from build123d import *

# Parameters (mm, degrees)
SKETCH1_R           = 12.15
SKETCH1_R_2         = 16.15
BOSS_EXTRUDE1_DEPTH = 5.4
FILLET1_R           = 30
CHAMFER1_SIZE       = 1
SKETCH2_R           = 14.75534968
SKETCH2_R_2         = 10
SKETCH2_R_3         = 19.025242353
SKETCH2_R_4         = 14
BOSS_EXTRUDE2_DEPTH = 0.6


with BuildPart() as part:
    # Sketch1 → Boss-Extrude1 (new body)
    with BuildSketch(Plane(origin=(0, 0, 0), x_dir=(1, 0, 0), z_dir=(0, 1, 0))):
        with BuildLine():
            Line((54.45294862, -21), (63.75, -21))
            ThreePointArc((63.75, -21), (84.75, 0), (63.75, 21))
            Line((63.75, 21), (54.45294862, 21))
            ThreePointArc((54.45294862, 21), (48.447855306, 13.72835863), (39.420454068, 11))
            Line((39.420454068, 11), (-39.420454068, 11))
            ThreePointArc((-39.420454068, 11), (-48.447855306, 13.72835863), (-54.45294862, 21))
            Line((-54.45294862, 21), (-63.75, 21))
            ThreePointArc((-63.75, 21), (-84.75, 0), (-63.75, -21))
            Line((-63.75, -21), (-54.45294862, -21))
            ThreePointArc((-54.45294862, -21), (-48.447855306, -13.72835863), (-39.420454068, -11))
            Line((-39.420454068, -11), (39.420454068, -11))
            ThreePointArc((39.420454068, -11), (48.447855306, -13.72835863), (54.45294862, -21))
        make_face()
        with Locations(Location((-63.75, 0, 0), (0, 0, 90))):
            Circle(SKETCH1_R, mode=Mode.SUBTRACT)
        with Locations(Location((63.75, 0, 0), (0, 0, 90))):
            Circle(SKETCH1_R_2, mode=Mode.SUBTRACT)
    extrude(amount=BOSS_EXTRUDE1_DEPTH)

    # Fillet1
    # the kernel refuses this fillet: 30 mm, written as the material it takes off along each edge
    with BuildSketch(Plane(origin=(-54.45294862, -23.24262845, -21), x_dir=(0.5987620470660618, 0, 0.8009269698251266), z_dir=(0, 1, 0))) as fillet1_piece_1:
        with BuildLine():
            CenterArc((15.193568911, -29.102905777), FILLET1_R, 104.047021464, 29.74238235)
            Line((-5.566721516, -7.44625919), (-5.981927325, -7.013126259))
            ThreePointArc((-5.981927325, -7.013126259), (-3.26391694, -3.363872367), (-0.480556182, 0.359257228))
            Line((-0.480556182, 0.359257228), (0.145630869, 0.582058116))
            ThreePointArc((0.145630869, 0.582058116), (3.95601272, 0.11261485), (7.76639457, 0.582058116))
            Line((7.76639457, 0.582058116), (7.912025439, 0))
        make_face()
    extrude(amount=51.885256901, mode=Mode.SUBTRACT)
    with BuildSketch(Plane(origin=(54.45294862, -23.24262845, -21), x_dir=(1, 0, 0), z_dir=(0, 1, 0)), Plane(origin=(-54.45294862, -23.24262845, 21), x_dir=(-1, 0, 0), z_dir=(0, 1, 0))) as fillet1_piece_2:
        with BuildLine():
            CenterArc((14.211969714, -29.594654547), FILLET1_R, 99.429309033, 29.74238235)
            Line((-4.737420548, -6.33695456), (-5.116408354, -5.87180056))
            ThreePointArc((-5.116408354, -5.87180056), (-2.458906545, -3.101047782), (-0.55338428, 0.231874618))
            Line((-0.55338428, 0.231874618), (0, 0.6))
            ThreePointArc((0, 0.6), (4.64852569, 0.6), (9.198753014, 0.591893091))
            Line((9.198753014, 0.591893091), (9.29705138, 0))
        make_face()
    extrude(amount=51.885256901, mode=Mode.SUBTRACT)
    with BuildSketch(Plane(origin=(54.45294862, -23.24262845, 21), x_dir=(1, 0, 0), z_dir=(0, 1, 0))) as fillet1_piece_3:
        with BuildLine():
            CenterArc((14.211969714, 29.594654547), FILLET1_R, 230.828308617, 29.74238235)
            Line((-4.737420548, 6.33695456), (-5.116408354, 5.87180056))
            ThreePointArc((-5.116408354, 5.87180056), (-2.458906545, 3.101047782), (-0.55338428, -0.231874618))
            Line((-0.55338428, -0.231874618), (0, -0.6))
            ThreePointArc((0, -0.6), (4.64852569, -0.6), (9.198753014, -0.591893091))
            Line((9.198753014, -0.591893091), (9.29705138, 0))
        make_face()
    extrude(amount=51.885256901, mode=Mode.SUBTRACT)

    # Chamfer1
    # the kernel refuses this chamfer: 1 mm, written as the material it takes off along each edge
    with BuildSketch(Plane(origin=(63.75, 5.4, 0), x_dir=(-0.12235070165055995, 0, 0.9924869297908239), z_dir=(-0.9924869297908239, 0, -0.12235070165055995))) as chamfer1_piece_1:
        Polygon((21, -CHAMFER1_SIZE), (21 - CHAMFER1_SIZE, 0), (21, 0), align=None)
    revolve(axis=Axis((63.75, 5.4, 0), (0, 1, 0)), revolution_arc=194.055575488, mode=Mode.SUBTRACT)
    with BuildSketch(Plane(origin=(39.420454068, 5.4, -27.298794623), x_dir=(0.6316463420707552, 0, 0.7752566662394039), z_dir=(0.7752566662394039, 0, -0.6316463420707552))) as chamfer1_piece_2:
        Polygon((16.298794623 + CHAMFER1_SIZE, 0), (16.298794623, CHAMFER1_SIZE), (16.298794623, 0), align=None)
    revolve(axis=Axis((39.420454068, 5.4, -27.298794623), (0, -1, 0)), revolution_arc=39.171691383, mode=Mode.SUBTRACT)
    with BuildSketch(Plane(origin=(39.420454068, 5.4, -11), x_dir=(0, 0, 1), z_dir=(-1, 0, 0)), Plane(origin=(-39.420454068, 5.4, 11), x_dir=(0, 0, -1), z_dir=(1, 0, 0))) as chamfer1_piece_3:
        Polygon((CHAMFER1_SIZE, 0), (0, -CHAMFER1_SIZE), (0, 0), align=None)
    extrude(amount=78.840908135, mode=Mode.SUBTRACT)
    with BuildSketch(Plane(origin=(-39.420454068, 5.4, -27.298794623), x_dir=(0, 0, 1), z_dir=(1, 0, 0))) as chamfer1_piece_4:
        Polygon((16.298794623 + CHAMFER1_SIZE, 0), (16.298794623, CHAMFER1_SIZE), (16.298794623, 0), align=None)
    revolve(axis=Axis((-39.420454068, 5.4, -27.298794623), (0, -1, 0)), revolution_arc=39.171691383, mode=Mode.SUBTRACT)
    with BuildSketch(Plane(origin=(39.420454068, 5.4, 27.298794623), x_dir=(0, 0, -1), z_dir=(-1, 0, 0))) as chamfer1_piece_5:
        Polygon((16.298794623 + CHAMFER1_SIZE, 0), (16.298794623, CHAMFER1_SIZE), (16.298794623, 0), align=None)
    revolve(axis=Axis((39.420454068, 5.4, 27.298794623), (0, -1, 0)), revolution_arc=39.171691383, mode=Mode.SUBTRACT)
    with BuildSketch(Plane(origin=(-68.664918334, 5.4, -8.594654547), x_dir=(0.6316463420707823, 0, 0.7752566662393817), z_dir=(0.7752566662393817, 0, -0.6316463420707823))) as chamfer1_piece_6:
        Polygon((30 - CHAMFER1_SIZE, 0), (30, CHAMFER1_SIZE), (30, 0), align=None)
    revolve(axis=Axis((-68.664918334, 5.4, -8.594654547), (0, -1, 0)), revolution_arc=44.477686757, mode=Mode.SUBTRACT)
    with BuildSketch(Plane(origin=(68.664918334, 5.4, -8.594654547), x_dir=(0.09247477859233537, 0, 0.9957150271660554), z_dir=(0.9957150271660554, 0, -0.09247477859233537))) as chamfer1_piece_7:
        Polygon((30, CHAMFER1_SIZE), (30 - CHAMFER1_SIZE, 0), (30, 0), align=None)
    revolve(axis=Axis((68.664918334, 5.4, -8.594654547), (0, -1, 0)), revolution_arc=44.477686757, mode=Mode.SUBTRACT)
    with BuildSketch(Plane(origin=(68.664918334, 5.4, 8.594654547), x_dir=(-0.6316463420707823, 0, -0.7752566662393817), z_dir=(-0.7752566662393817, 0, 0.6316463420707823))) as chamfer1_piece_8:
        Polygon((30, CHAMFER1_SIZE), (30 - CHAMFER1_SIZE, 0), (30, 0), align=None)
    revolve(axis=Axis((68.664918334, 5.4, 8.594654547), (0, -1, 0)), revolution_arc=44.477686757, mode=Mode.SUBTRACT)
    with BuildSketch(Plane(origin=(-68.664918334, 5.4, 8.594654547), x_dir=(-0.09247477859236329, 0, -0.9957150271660529), z_dir=(-0.9957150271660529, 0, 0.09247477859236329))) as chamfer1_piece_9:
        Polygon((30 - CHAMFER1_SIZE, 0), (30, CHAMFER1_SIZE), (30, 0), align=None)
    revolve(axis=Axis((-68.664918334, 5.4, 8.594654547), (0, -1, 0)), revolution_arc=44.477686757, mode=Mode.SUBTRACT)
    with BuildSketch(Plane(origin=(-63.75, 5.4, 0), x_dir=(0.12235070165055861, 0, -0.992486929790824), z_dir=(0.992486929790824, 0, 0.12235070165055861))) as chamfer1_piece_10:
        Polygon((21 - CHAMFER1_SIZE, 0), (21, -CHAMFER1_SIZE), (21, 0), align=None)
    revolve(axis=Axis((-63.75, 5.4, 0), (0, 1, 0)), revolution_arc=194.055575488, mode=Mode.SUBTRACT)
    with BuildSketch(Plane(origin=(-39.420454068, 5.4, 27.298794623), x_dir=(-0.6316463420707533, 0, -0.7752566662394053), z_dir=(-0.7752566662394053, 0, 0.6316463420707533))) as chamfer1_piece_11:
        Polygon((16.298794623 + CHAMFER1_SIZE, 0), (16.298794623, CHAMFER1_SIZE), (16.298794623, 0), align=None)
    revolve(axis=Axis((-39.420454068, 5.4, 27.298794623), (0, -1, 0)), revolution_arc=39.171691383, mode=Mode.SUBTRACT)
    with BuildSketch(Plane(origin=(-63.75, 5.4, 0), x_dir=(0, 0, -1), z_dir=(1, 0, 0))) as chamfer1_piece_12:
        Polygon((12.15 + CHAMFER1_SIZE, 0), (12.15, -CHAMFER1_SIZE), (12.15, 0), align=None)
    revolve(axis=Axis((-63.75, 5.4, 0), (0, 1, 0)), mode=Mode.SUBTRACT)
    with BuildSketch(Plane(origin=(63.75, 5.4, 0), x_dir=(0, 0, -1), z_dir=(1, 0, 0))) as chamfer1_piece_13:
        Polygon((16.15 + CHAMFER1_SIZE, 0), (16.15, -CHAMFER1_SIZE), (16.15, 0), align=None)
    revolve(axis=Axis((63.75, 5.4, 0), (0, 1, 0)), mode=Mode.SUBTRACT)

    # Sketch2 → Boss-Extrude2 (add)
    # profile 1 of 2: a face of its own
    with BuildSketch(Plane.XZ):
        with Locations((-63.75, 0)):
            Circle(SKETCH2_R)
        with Locations(Location((-63.75, 0, 0), (0, 0, 270))):
            Circle(SKETCH2_R_2, mode=Mode.SUBTRACT)
    # profile 2 of 2: a face of its own
    with BuildSketch(Plane.XZ):
        with Locations((63.75, 0)):
            Circle(SKETCH2_R_3)
        with Locations(Location((63.75, 0, 0), (0, 0, 270))):
            Circle(SKETCH2_R_4, mode=Mode.SUBTRACT)
    extrude(amount=-BOSS_EXTRUDE2_DEPTH)


solid = part.part
Design review of the part built by this model. Coordinates are the model's own, in mm. A direction names the side the tool comes from. Round coordinates to 2 decimals unless told otherwise and drop trailing zeros. Order: outer loops, then holes, each group sorted by start corner. A loop starts at its lowest first (then second) coordinate and runs counter-clockwise, first axis right, second up. Notation, with made-up numbers: M 75,-14.5 L 93,-14.5 A33 ccw 93,13.5 Z; hole C 64,78.5 d10. An arc over 180 degrees is marked long. Answer as CSV lines item,"result". Start each with the question number.
1) Wall thickness on line 1 along X through (y, z) = (0.55, 0); line 2 along X through (y, z) = (1.7, -8.5); line 3 along Z through (x, y) = (63.75, 1.9): over which ranges is each line inside the solid? List them lowest first. Write a range as [from, to].
2) The part is to be moulded in two halves that separate along Z. For faces 5 (the face through (-56.419, 2.169, 18.792)), 6 (the face through (-20, 0, 0)), 7 (the face through (83.905, 5.24, 0.443)), 8 (the face through (-73.995, 2.473, -6.532)), say which applies: +Z half, -Z half, draft (parallel to the pull), parting line (faces both ways), or undercut.
3) For pin 1 Ø1 at (x, y) = (13.5, 4.5) entering from +Z; pin 2 Ø1 at (x, y) = (3, 2.5) entering from -Z; pin 3 Ø1 at (y, z) = (3.5, -8) entering from -X, all flat-tipped, find the tip position at first contact; note any pin that passes through.
4) Add section B-B (y = 2). Give the boundary of the cut face in (x, z), then the cut area to 3 significant figures.
5) Add section A-A (z = 0). Give the boundary of the cut face in (x, y), then the cut area to 3 significant figures.
6) Add section C-C (x = 23). Give the boundary of the cut face in (y, z).
7) Tool access review of faces 1 (the face through (-83.919, 5.226, -0.444)), 2 (the face through (63.7, 0.6, 14.4)), 3 (the face through (56.419, 2.169, -18.792)), 4 (the face through (56.22, 2.169, 18.702)): name each direction out of +Z, -Z, +X, -X, +Y, -Y from which nothing blocks a thin tool from reaching the whole face with its end or side.
8) Add section D-D (z = 8.5). Give the number of separate pieces and of enclosed holes in the cut face, then the cut area to 3 significant figures.
Resolved:
1,line 1,"[-84.75, -73.75], [-53.75, 49.75], [77.75, 84.75]"
1,line 2,"[-82.95, -72.43], [-55.07, 50.02], [77.48, 82.95]"
1,line 3,"[-21, -16.15], [16.15, 21]"
2,face 5,"+Z half"
2,face 6,"draft"
2,face 7,"parting line"
2,face 8,"undercut"
3,pin 1,"z = 11"
3,pin 2,"z = -11"
3,pin 3,"x = -83.37"
4,outline,"M -63.75,-21 A30 ccw -49.72,-14.66 A16.3 cw -39.42,-11 L 39.42,-11 A16.3 cw 49.72,-14.66 A30 ccw 63.75,-21 A21 ccw 63.75,21 A30 ccw 49.72,14.66 A16.3 cw 39.42,11 L -39.42,11 A16.3 cw -49.72,14.66 A30 ccw -63.75,21 A21 ccw Z; hole C -63.75,0 d24.3; hole C 63.75,0 d32.3"
4,area,"3,380 mm^2"
5,outline,"M -84.75,0 L -73.75,0 L -73.75,0.6 L -75.9,0.6 L -75.9,4.4 L -76.9,5.4 L -83.75,5.4 L -84.75,4.4 Z; M -53.75,0 L 49.75,0 L 49.75,0.6 L 47.6,0.6 L 47.6,4.4 L 46.6,5.4 L -50.6,5.4 L -51.6,4.4 L -51.6,0.6 L -53.75,0.6 Z; M 77.75,0 L 84.75,0 L 84.75,4.4 L 83.75,5.4 L 80.9,5.4 L 79.9,4.4 L 79.9,0.6 L 77.75,0.6 Z"
5,area,"612 mm^2"
6,outline,"M 0,-11 L 4.4,-11 L 5.4,-10 L 5.4,10 L 4.4,11 L 0,11 Z"
7,face 1,"-X, +Y"
7,face 2,"+Y"
7,face 3,"-Z, +Y, -Y"
7,face 4,"+Z, +Y, -Y"
8,separate pieces,"3"
8,enclosed holes,"0"
8,area,"657 mm^2"
